Geometry: final body of the model. Coordinates: model frame, mm. A direction names the side the tool comes from. Give positions to 0.01 mm unless a question says otherwise; leave off trailing zeros. Loops run counter-clockwise (first coordinate to the right, second up) from the corner with the lowest first, then second, coordinate; pieces in that order, holes last.
Autodesk Inventor part; units mm, degrees
ref_plane "YZ Plane" through (0, 0, 0) normal (1, 0, 0) x (0, 1, 0)
ref_plane "XZ Plane" through (0, 0, 0) normal (0, 1, 0) x (-1, 0, 0)
ref_plane "XY Plane" through (0, 0, 0) normal (0, 0, 1) x (1, 0, 0)
sketch "Boceto1" plane through (0, 0, 0) normal (0, 0, 1) x (1, 0, 0)
  line L0 (0, 0) -> (60, 0)
  line L1 (60, 0) -> (60, 20)
  line L2 (60, 20) -> (0, 20)
  line L3 (0, 20) -> (0, 0)
  line L4 (30, 20) -> (10.5, 20)
  line L5 (30, 20) -> (49.5, 20)
  line L6 (49.5, 20) -> (49.5, 10)
  circle A0 centre (10.5, 10) radius 1.5
  circle A1 centre (49.5, 10) radius 1.5
  line L7 (30, 20) -> (35, 20)
  line L8 (35, 20) -> (35, 10)
  line L9 (38, 10) -> (38, 12)
  line L10 (38, 10) -> (38, 8)
  line L11 (38, 8) -> (35, 8)
  line L12 (35, 8) -> (35, 10)
  line L13 (38, 12) -> (35, 12)
  line L14 (30, 20) -> (25, 20)
  line L15 (25, 20) -> (25, 12)
  line L16 (25, 12) -> (25, 8)
  line L17 (25, 8) -> (22, 8)
  line L18 (22, 8) -> (22, 12)
  line L19 (22, 12) -> (25, 12)
  dimension "d0" = 60
  dimension "d1" = 20
  dimension "d2" = 19.5
  dimension "d3" = 19.5
  dimension "d4" = 10
  dimension "d5" = 3
  dimension "d6" = 3
  dimension "d7" = 5
  dimension "d8" = 3
  dimension "d9" = 2
  dimension "d10" = 2
  dimension "d11" = 5
  dimension "d12" = 3
extrude "Extrusión1" add sketch "Boceto1" along normal blind 3
fillet "Empalme1" radius 2 4 edges at (60, 20, 1.5) (60, 0, 1.5) (0, 20, 1.5) (0, 0, 1.5)
fillet "Empalme2" radius 1 8 edges at (0.5858, 19.4142, 3) (0, 10, 3) (0.5858, 0.5858, 3) (30, 0, 3) (59.4142, 0.5858, 3) (60, 10, 3) (59.4142, 19.4142, 3) (42.25, 20, 3)
properties part number "tapa_soporte_bateria"
Item 1: Section query A-A on y = 10. Return loops of the section in (x, z).
Values follow:
outline: (0, 0) - (9, 0) - (9, 3) - (1, 3) arc R1 ccw to (0, 2) - close; (12, 0) - (22, 0) - (22, 3) - (12, 3) - close; (25, 0) - (35, 0) - (35, 3) - (25, 3) - close; (38, 0) - (48, 0) - (48, 3) - (38, 3) - close; (51, 0) - (60, 0) - (60, 2) arc R1 ccw to (59, 3) - (51, 3) - close
Item 2: Section query C-C on x = 36. Return loops of the section in (y, z).
Values follow:
outline: (0, 0) - (8, 0) - (8, 3) - (1, 3) arc R1 ccw to (0, 2) - close; (12, 0) - (20, 0) - (20, 2) arc R1 ccw to (19, 3) - (12, 3) - close
Item 3: Draft query along X for faces 1 (the face through (0.285, 10.112, 2.699)), 2 (the face through (37, 12, 1)), 3 (the face through (59.4, 0.57, 1.01)), 4 (the face through (9.3, 10.9, 1.5)). Return one class per face: +X half, -X half, draft (parallel to the pull), parting line (faces both ways), or undercut.
Values follow:
face 1: -X half
face 2: undercut
face 3: +X half
face 4: undercut
Item 4: Pin query (flat end, axial travel): pin 1 (2.5 mm diameter, centred on x = 10.5, y = 10, fed in from +Z). Return the tip coordinate at first contact, or that it passes through.
Values follow:
pin 1: passes through
Item 5: Set-up query: faces 5 (the face through (59.715, 9.888, 2.699)), 6 (the face through (37, 8, 1)). Return all of +Z, -Z, +X, -X, +Y, -Y with unobstructed straight access to the full face (end or side cutting, diameter ignored); none if empty.
Values follow:
face 5: +Z, +X, +Y, -Y
face 6: +Z, -Z
Item 6: Section query B-B on z = 0.7. Return loops of the section in (x, y).
Values follow:
outline: (0, 2) arc R2 ccw to (2, 0) - (58, 0) arc R2 ccw to (60, 2) - (60, 18) arc R2 ccw to (58, 20) - (2, 20) arc R2 ccw to (0, 18) - close; hole circle Ø3 at (10.5, 10); hole (22, 8) - (25, 8) - (25, 12) - (22, 12) - close; hole (35, 8) - (38, 8) - (38, 12) - (35, 12) - close; hole circle Ø3 at (49.5, 10)
Item 7: Ray query, probe 1 along Y at (x, z) = (22.5, 1.65); probe 2 along Y at (x, z) = (49.5, 1); probe 3 along X at (y, z) = (8.75, 0.55). Return the intervals inside material, ascending.
Values follow:
probe 1: y = 0 to 8, 12 to 20
probe 2: y = 0 to 8.5, 11.5 to 20
probe 3: x = 0 to 9.67, 11.33 to 22, 25 to 35, 38 to 48.67, 50.33 to 60
Item 8: Section query D-D on x = 49.5. Return loops of the section in (y, z), plus the area to 3 significant figures.
Values follow:
outline: (0, 0) - (8.5, 0) - (8.5, 3) - (1, 3) arc R1 ccw to (0, 2) - close; (11.5, 0) - (20, 0) - (20, 2) arc R1 ccw to (19, 3) - (11.5, 3) - close
area: 50.6 mm2
